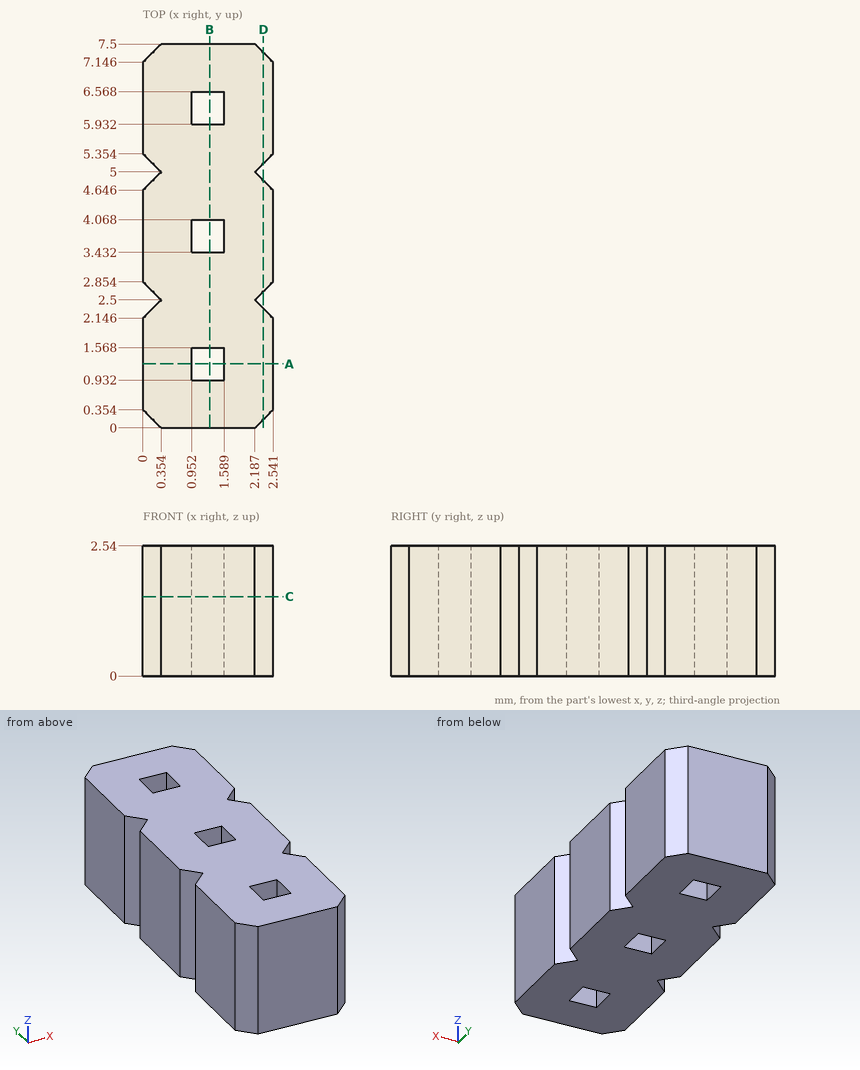
The figure shows three views and two pictorial views of one solid part (mm, origin at its lowest corner). Answer the questions. Round coordinates to 2 decimals unless told otherwise and drop trailing zeros. Write each loop counter-clockwise with the first axis right and the second up, starting at its lowest first coordinate (ties: lowest second). Pieces come first, ordered by that corner, then holes. Notation, with made-up numbers: (15.25, 69.5) - (57.25, 69.5) arc R21 cw to (57.25, 100.5) - close; hole circle Ø11 at (31.5, 46). An arc over 180 degrees is marked (long way). Answer in a Markdown table with one row per item. Add a question column.
1. A cutting plane is placed at A-A, the plane y = 1.25. Determine the outline of the cut face in (x, z).
2. Find the intervals of material crossed by line 1 along Y through (x, z) = (1.45, 2.45); line 2 along X through (y, z) = (1, 0.4); line 3 along Y through (x, z) = (0.25, 1.05) (1 decimal), in increasing order. Write a range as from..to.
3. A cutting plane is placed at B-B, the plane x = 1.3. Determine the outline of the cut face in (y, z), and give its area (3 significant figures).
4. A cutting plane is placed at C-C, the plane z = 1.55. Count the separate pieces of the cut face and the enclosed holes in it, and give its area (3 significant figures).
5. A cutting plane is placed at D-D, the plane x = 2.35. Determine the outline of the cut face in (y, z).
Worked out:
| question | item | result |
|---|---|---|
| 1 | outline | (0, 0) - (0.95, 0) - (0.95, 2.54) - (0, 2.54) - close; (1.59, 0) - (2.54, 0) - (2.54, 2.54) - (1.59, 2.54) - close |
| 2 | line 1 | 0..0.93, 1.57..3.43, 4.07..5.93, 6.57..7.5 |
| 2 | line 2 | 0..0.95, 1.59..2.54 |
| 2 | line 3 | 0.1..2.4, 2.6..4.9, 5.1..7.4 |
| 3 | outline | (0, 0) - (0.93, 0) - (0.93, 2.54) - (0, 2.54) - close; (1.57, 0) - (3.43, 0) - (3.43, 2.54) - (1.57, 2.54) - close; (4.07, 0) - (5.93, 0) - (5.93, 2.54) - (4.07, 2.54) - close; (6.57, 0) - (7.5, 0) - (7.5, 2.54) - (6.57, 2.54) - close |
| 3 | area | 14.2 mm^2 |
| 4 | separate pieces | 1 |
| 4 | enclosed holes | 3 |
| 4 | area | 17.1 mm^2 |
| 5 | outline | (0.16, 0) - (2.34, 0) - (2.34, 2.54) - (0.16, 2.54) - close; (2.66, 0) - (4.84, 0) - (4.84, 2.54) - (2.66, 2.54) - close; (5.16, 0) - (7.34, 0) - (7.34, 2.54) - (5.16, 2.54) - close |
